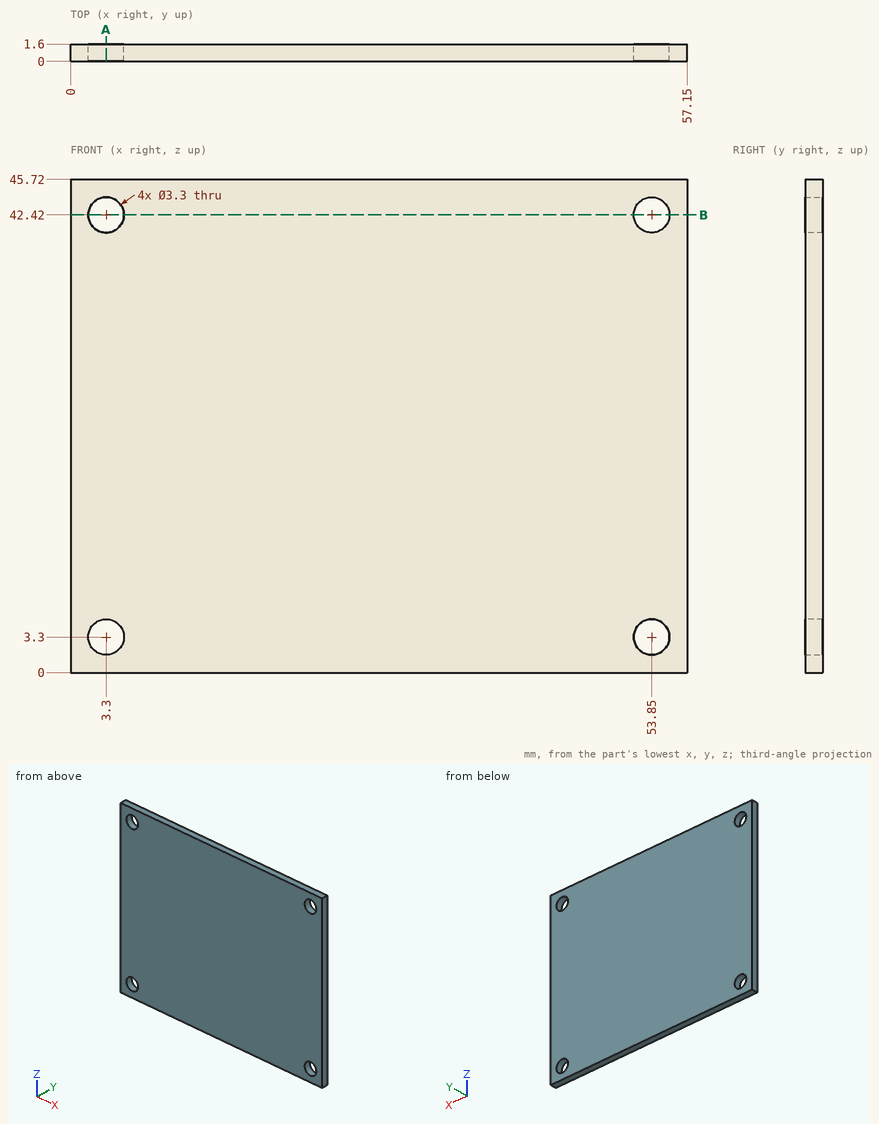
The drawing under review shows one solid part. Ordinate dimensions are in mm from its lowest x, y, z. Give positions to 0.01 mm unless a question says otherwise; leave off trailing zeros. Order: outer loops, then holes, each group sorted by start corner. A loop starts at its lowest first (then second) coordinate and runs counter-clockwise, first axis right, second up. Notation, with made-up numbers: (21, 86) - (64, 86) arc R10 ccw to (64, 100) - close; hole circle Ø10 at (71.25, 22). An arc over 180 degrees is marked (long way). Answer as a JSON object with one key per item and string values. Group by question number.
Item 1: Wall thickness on line 1 along Z through (x, y) = (53.85, 0.75); line 2 along X through (y, z) = (0.9, 3.3); line 3 along X through (y, z) = (0.85, 4): over which ranges is each line inside the solid? List them lowest first.
Item 2: Take a section at A-A on x = 3.3. Give the boundary of the cut face in (y, z), and give its area (3 significant figures).
Item 3: Take a section at B-B on z = 42.42. Give the boundary of the cut face in (x, y).
Reported:
{
 "1": {"line 1": "0 to 1.65, 4.95 to 40.77, 44.07 to 45.72", "line 2": "0 to 1.65, 4.95 to 52.2, 55.5 to 57.15", "line 3": "0 to 1.81, 4.79 to 52.36, 55.34 to 57.15"},
 "2": {"outline": "(0, 0) - (1.6, 0) - (1.6, 1.65) - (0, 1.65) - close; (0, 4.95) - (1.6, 4.95) - (1.6, 40.77) - (0, 40.77) - close; (0, 44.07) - (1.6, 44.07) - (1.6, 45.72) - (0, 45.72) - close", "area": "62.6 mm^2"},
 "3": {"outline": "(0, 0) - (1.65, 0) - (1.65, 1.6) - (0, 1.6) - close; (4.95, 0) - (52.2, 0) - (52.2, 1.6) - (4.95, 1.6) - close; (55.5, 0) - (57.15, 0) - (57.15, 1.6) - (55.5, 1.6) - close"}
}
